from build123d import *

# Parameters (mm, degrees)
BOSS_EXTRUDE1_DEPTH     = 20
FILLET1_R               = 4
SKETCH2_R               = 2.75
CUT_EXTRUDE1_DEPTH      = 1.5
LPATTERN1_COUNT         = 2
LPATTERN1_PITCH         = 30
CUT_EXTRUDE2_DEPTH      = 29.722813233
CUT_EXTRUDE2_DEPTH_BACK = 29.722813233
WRAP1_DEPTH             = 1


# Read off the part's stored shape, not the designer's step: Wrap1
with BuildPart() as part:
    # Sketch1 → Boss-Extrude1 (new body)
    with BuildSketch(Plane(origin=(0, 0, 0), x_dir=(1, 0, 0), z_dir=(0, 1, 0))):
        with BuildLine():
            Line((15, -5), (-15, -5))
            ThreePointArc((-15, -5), (-20, 0), (-15, 5))
            Line((-15, 5), (15, 5))
            ThreePointArc((15, 5), (20, 0), (15, -5))
        make_face()
    extrude(amount=BOSS_EXTRUDE1_DEPTH)

    # Fillet1
    fillet1_edges = [part.edges().sort_by_distance(p)[0] for p in [
        (-20, 20, 0),
        (0, 20, 5),
        (20, 20, 0),
        (0, 20, -5),
    ]]
    fillet(fillet1_edges, radius=FILLET1_R)

    # Sketch2 → Cut-Extrude1 (cut)
    with BuildSketch(Plane.XZ):
        with Locations(Location((-15, 0, 0), (0, 0, 270))):
            Circle(SKETCH2_R)
    cut_extrude1 = extrude(amount=-CUT_EXTRUDE1_DEPTH, mode=Mode.SUBTRACT)

    # LPattern1: Cut-Extrude1 ×2
    with Locations(*[(i * LPATTERN1_PITCH, 0, 0) for i in range(1, LPATTERN1_COUNT)]):
        add(cut_extrude1, mode=Mode.SUBTRACT)

    # Sketch3 → Cut-Extrude2 (cut, two sides: drawn at the far end of the back side and taken through both)
    with BuildSketch(Plane.XY.offset(-CUT_EXTRUDE2_DEPTH_BACK)):
        with BuildLine():
            Line((-5, 23), (5, 23))
            ThreePointArc((5, 23), (8, 20), (5, 17))
            Line((5, 17), (-5, 17))
            ThreePointArc((-5, 17), (-8, 20), (-5, 23))
        make_face()
    extrude(amount=CUT_EXTRUDE2_DEPTH + CUT_EXTRUDE2_DEPTH_BACK, mode=Mode.SUBTRACT)

    # Wrap1 outline → Wrap1 (add)
    with BuildSketch(Plane(origin=(0, 17, 0), x_dir=(1, 0, 0), z_dir=(0, 1, 0))):
        with BuildLine():
            add(Edge.make_bspline(
                [(0.968558604, -2.112404227), (1.023340463, -2.110381468), (1.128135866, -2.106512015), (1.275421614, -2.065066433), (1.40411806, -1.999153831), (1.494113345, -1.918796765), (1.555259283, -1.8377784), (1.600182088, -1.761379971), (1.643056037, -1.669468115), (1.68410688, -1.562162987), (1.724115658, -1.439672484), (1.762787282, -1.301883834), (1.796828359, -1.147944523), (1.819117415, -1.040313742), (1.830738091, -0.984199098)],
                knots=[0, 0, 0, 0, 0.10403341, 0.199011557, 0.288612319, 0.377191825, 0.425797175, 0.481425289, 0.545557079, 0.61863331, 0.699984683, 0.790771883, 0.890916323, 1, 1, 1, 1], degree=3))
            Line((0.968558604, -2.112404227), (-1.502595242, -2.112404227))
            add(Edge.make_bspline(
                [(0.359584245, -0.57875038), (0.287589412, -0.631266446), (0.149119993, -0.732271876), (-0.052040125, -0.874957595), (-0.232151558, -1.010570949), (-0.396984875, -1.13231455), (-0.543079134, -1.243803459), (-0.672030163, -1.343433338), (-0.782764208, -1.43141572), (-0.961872458, -1.579798827), (-1.207220157, -1.798528227), (-1.40469562, -2.00837263), (-1.502595242, -2.112404227)],
                knots=[0, 0, 0, 0, 0.110593572, 0.212707314, 0.306051588, 0.390379305, 0.467018215, 0.534117187, 0.592614819, 0.642525788, 0.822780058, 1, 1, 1, 1], degree=3))
            add(Edge.make_bspline(
                [(2.103173989, 1.329903466), (2.066781163, 1.246346618), (1.99482956, 1.081147874), (1.86047631, 0.847661593), (1.71297016, 0.626020413), (1.571074283, 0.452909604), (1.445054335, 0.315568643), (1.334068385, 0.207346612), (1.208958187, 0.091994137), (1.069166496, -0.030104), (0.913592831, -0.158279882), (0.741560734, -0.29208501), (0.556771712, -0.435146764), (0.42660857, -0.529939289), (0.359584245, -0.57875038)],
                knots=[0, 0, 0, 0, 0.10413489, 0.205883221, 0.307528832, 0.408265615, 0.461433854, 0.520606469, 0.585444086, 0.656004792, 0.732803839, 0.815893726, 0.905198979, 1, 1, 1, 1], degree=3))
            add(Edge.make_bspline(
                [(2.258622707, 2.155223979), (2.256854974, 2.081406691), (2.253395008, 1.936924834), (2.223825952, 1.724789841), (2.174767432, 1.522306219), (2.126875674, 1.393600214), (2.103173989, 1.329903466)],
                knots=[0, 0, 0, 0, 0.261979501, 0.512769921, 0.758869279, 1, 1, 1, 1], degree=3))
            add(Edge.make_bspline(
                [(-0.061890114, 4.14400603), (0.022564629, 4.141920306), (0.18812583, 4.13783155), (0.430620451, 4.112847977), (0.660471364, 4.067558501), (0.878305178, 4.005888588), (1.082018473, 3.923000729), (1.274759097, 3.825795699), (1.453280397, 3.707304776), (1.618929442, 3.573545968), (1.768923738, 3.427244365), (1.900049838, 3.270535022), (2.011299511, 3.105351175), (2.101257211, 2.93081783), (2.172841542, 2.749020464), (2.221753805, 2.558426678), (2.253872753, 2.359840276), (2.257020026, 2.224263519), (2.258622707, 2.155223979)],
                knots=[0, 0, 0, 0, 0.074102612, 0.14526736, 0.21355926, 0.279416432, 0.343556942, 0.406228654, 0.468492489, 0.531146675, 0.592790073, 0.652016559, 0.710119813, 0.767135501, 0.823967905, 0.881147087, 0.939476717, 1, 1, 1, 1], degree=3))
            add(Edge.make_bspline(
                [(-1.906441396, 3.445288081), (-1.848306189, 3.501112989), (-1.732554849, 3.612264359), (-1.538609793, 3.754854821), (-1.330466242, 3.876473687), (-1.105791254, 3.973994027), (-0.866480346, 4.051164268), (-0.611446439, 4.105367467), (-0.341562002, 4.137488539), (-0.156530269, 4.14180053), (-0.061890114, 4.14400603)],
                knots=[0, 0, 0, 0, 0.119107626, 0.23715177, 0.355050392, 0.47498588, 0.598670295, 0.726365388, 0.860041186, 1, 1, 1, 1], degree=3))
            add(Edge.make_bspline(
                [(-2.459326011, 2.031826543), (-2.458122329, 2.10083777), (-2.455751672, 2.236755643), (-2.42704922, 2.435648535), (-2.383831572, 2.625974396), (-2.325084873, 2.808678323), (-2.245799792, 2.981581962), (-2.150493697, 3.146407777), (-2.038697096, 3.303051555), (-1.950794522, 3.397587797), (-1.906441396, 3.445288081)],
                knots=[0, 0, 0, 0, 0.132803649, 0.26155729, 0.386082589, 0.508400008, 0.630401232, 0.751619273, 0.874674186, 1, 1, 1, 1], degree=3))
            add(Edge.make_bspline(
                [(-1.520223447, 0.759390645), (-1.585420599, 0.763118791), (-1.713143024, 0.770422298), (-1.895082142, 0.836934937), (-2.058691576, 0.943915448), (-2.201841078, 1.092044894), (-2.320121913, 1.277705611), (-2.399559254, 1.501224402), (-2.452612405, 1.75530448), (-2.457009968, 1.936432658), (-2.459326011, 2.031826543)],
                knots=[0, 0, 0, 0, 0.110139331, 0.215764983, 0.323707128, 0.438906263, 0.562183724, 0.693638164, 0.838649921, 1, 1, 1, 1], degree=3))
            add(Edge.make_bspline(
                [(-0.613172165, 1.631185517), (-0.616054345, 1.570486701), (-0.621662157, 1.45238594), (-0.671323685, 1.283175242), (-0.754629801, 1.131365188), (-0.869218028, 1.000302814), (-1.00648217, 0.893380798), (-1.162575656, 0.81342959), (-1.336719307, 0.768952542), (-1.458017598, 0.762632021), (-1.520223447, 0.759390645)],
                knots=[0, 0, 0, 0, 0.129242333, 0.251464839, 0.372304265, 0.495878621, 0.620081591, 0.741344555, 0.867352775, 1, 1, 1, 1], degree=3))
            add(Edge.make_bspline(
                [(-1.273428575, 2.371570132), (-1.221111857, 2.356431424), (-1.121681232, 2.327659528), (-0.986315759, 2.264054818), (-0.872118751, 2.188748181), (-0.775565412, 2.103031066), (-0.702763657, 2.001965174), (-0.650977929, 1.888692008), (-0.61737495, 1.763975364), (-0.614599413, 1.676280399), (-0.613172165, 1.631185517)],
                knots=[0, 0, 0, 0, 0.151156851, 0.287281401, 0.413669873, 0.530293514, 0.644009236, 0.756908248, 0.874996313, 1, 1, 1, 1], degree=3))
            add(Edge.make_bspline(
                [(-1.659646524, 2.52701885), (-1.641908981, 2.5134804), (-1.599762076, 2.48131113), (-1.513799429, 2.446453071), (-1.403911325, 2.405291879), (-1.319666952, 2.383519902), (-1.273428575, 2.371570132)],
                knots=[0, 0, 0, 0, 0.159109439, 0.378066483, 0.65864549, 1, 1, 1, 1], degree=3))
            add(Edge.make_bspline(
                [(-1.741377293, 2.725736799), (-1.740702967, 2.705828636), (-1.739402264, 2.667427893), (-1.722346439, 2.613602242), (-1.696843256, 2.565494988), (-1.672067897, 2.539867464), (-1.659646524, 2.52701885)],
                knots=[0, 0, 0, 0, 0.268945253, 0.518766978, 0.758729042, 1, 1, 1, 1], degree=3))
            add(Edge.make_bspline(
                [(-0.509005498, 3.631185517), (-0.593702292, 3.627478268), (-0.757485819, 3.620309328), (-0.992510379, 3.565399378), (-1.204920463, 3.4708981), (-1.388970755, 3.342097951), (-1.54050767, 3.195942921), (-1.655393233, 3.044422755), (-1.727025811, 2.886507887), (-1.736695124, 2.778188345), (-1.741377293, 2.725736799)],
                knots=[0, 0, 0, 0, 0.151816317, 0.293576777, 0.429964406, 0.566304914, 0.694365033, 0.806085808, 0.906100976, 1, 1, 1, 1], degree=3))
            add(Edge.make_bspline(
                [(0.617597066, 2.220929107), (0.616798314, 2.277062503), (0.615251229, 2.385786079), (0.599863671, 2.542997259), (0.579004071, 2.690242583), (0.544058374, 2.826348498), (0.504153512, 2.954009696), (0.449772713, 3.069509609), (0.389899195, 3.176431124), (0.318093883, 3.271087373), (0.240513737, 3.356936451), (0.152380296, 3.428872442), (0.059506725, 3.491963217), (-0.040243661, 3.543993611), (-0.147906764, 3.581901434), (-0.261368703, 3.611540097), (-0.38306343, 3.626855058), (-0.466235221, 3.629714881), (-0.509005498, 3.631185517)],
                knots=[0, 0, 0, 0, 0.082284271, 0.159374645, 0.231497254, 0.300083139, 0.36523236, 0.427274673, 0.486932074, 0.544586116, 0.60112786, 0.656190593, 0.710940404, 0.765594865, 0.820607428, 0.877984079, 0.93725451, 1, 1, 1, 1], degree=3))
            add(Edge.make_bspline(
                [(0.205738091, 0.635993209), (0.238640814, 0.700768661), (0.303861654, 0.829168655), (0.385865127, 1.026897746), (0.459663901, 1.22391557), (0.516579645, 1.422967903), (0.561905142, 1.621957205), (0.593823909, 1.82108009), (0.613938148, 2.020726724), (0.616375849, 2.154108657), (0.617597066, 2.220929107)],
                knots=[0, 0, 0, 0, 0.131745637, 0.261150462, 0.388067803, 0.513189353, 0.636374668, 0.758087597, 0.878808958, 1, 1, 1, 1], degree=3))
            add(Edge.make_bspline(
                [(-1.116377293, -1.107596534), (-1.03496234, -1.013767374), (-0.878016077, -0.832889839), (-0.655626445, -0.569536189), (-0.456135085, -0.32390871), (-0.280159151, -0.096566641), (-0.125247461, 0.111659158), (0.00577288, 0.302221735), (0.116680709, 0.473318508), (0.177475044, 0.584367138), (0.205738091, 0.635993209)],
                knots=[0, 0, 0, 0, 0.170005554, 0.327725258, 0.471696803, 0.603008639, 0.721148947, 0.826797124, 0.919478664, 1, 1, 1, 1], degree=3))
            add(Edge.make_bspline(
                [(-2.664454216, -3.057917047), (-2.628698989, -3.000910883), (-2.55158858, -2.877970296), (-2.41479269, -2.688825323), (-2.259314405, -2.474715573), (-2.074551732, -2.243606397), (-1.870318919, -1.988170585), (-1.640593125, -1.712928149), (-1.387471618, -1.416348269), (-1.20904993, -1.213142224), (-1.116377293, -1.107596534)],
                knots=[0, 0, 0, 0, 0.080973991, 0.174630064, 0.280853316, 0.39944862, 0.530692677, 0.674513651, 0.830941638, 1, 1, 1, 1], degree=3))
            Line((-2.664454216, -3.057917047), (-2.664454216, -3.548301662))
            Line((-2.664454216, -3.548301662), (2.156058604, -3.548301662))
            Line((2.156058604, -3.548301662), (2.361186809, -0.984199098))
            Line((2.361186809, -0.984199098), (1.830738091, -0.984199098))
        make_face()
    extrude(amount=WRAP1_DEPTH)


solid = part.part
Work out the finished part from the listing and answer in its coordinate system (mm). A direction names the side the tool comes from. Coordinates: 2 decimals unless noted, no trailing zeros. Loops run counter-clockwise (first coordinate to the right, second up) from the corner with the lowest first, then second, coordinate; pieces in that order, holes last. Notation, with made-up numbers: (80, 20) -> (132, 20) arc R16 ccw to (132, 35) -> close; hole circle Ø10 at (-33.75, -20.5). An arc over 180 degrees is marked (long way). Answer as CSV lines item,"result".
1) The part is cut by section C-C (x = 13.5). Give the vertices of the cut face in (y, z), and give its area (3 significant figures).
A:
outline,"(0, -5) -> (16, -5) arc R4 ccw to (20, -1) -> (20, 1) arc R4 ccw to (16, 5) -> (0, 5) -> (0, 2.3) -> (1.5, 2.3) -> (1.5, -2.3) -> (0, -2.3) -> close"
area,"186 mm²"
2) Flat-ended cylindrical pins translate along their axes: pin 1 (0.8 mm diameter, centred on x = -0.5, y = 17.5, fed in from -Z); pin 2 (3.5 mm diameter, centred on x = 15, z = 0, fed in from -Y); pin 3 (1.5 mm diameter, centred on y = 8.5, z = -2, fed in from -X). Find the tip coordinate at first contact, or state that the pin passes through.
A:
pin 1,"stops at z = -4.14"
pin 2,"stops at y = 1.5"
pin 3,"stops at x = -19.84"
3) Straight lines are drawn through the part: probe 1 along X at (y, z) = (1.1, 0); probe 2 along Y at (x, z) = (3.5, -3.25); probe 3 along X at (y, z) = (11.75, -0.25). For each, find the intervals that lie inside material, in ascending order.
A:
probe 1,"x = -20 to -17.75, -12.25 to 12.25, 17.75 to 20"
probe 2,"y = 0 to 17"
probe 3,"x = -19.99 to 19.99"
4) For a pull along X with two mould halves and no side action, classify faces 6 (the face through (2.257, 17.493, 2.284)), 7 (the face through (0, 0, 0)), 8 (the face through (20, 8, 0)) as released by +X, released by -X, zero draft, split by the parting line, or undercut.
A:
face 6,"undercut"
face 7,"zero draft"
face 8,"released by +X"
5) The part is cut by section A-A (x = -5.5). Give the vertices of the cut face in (y, z).
A:
outline,"(0, -5) -> (16, -5) arc R4 ccw to (17.04, -4.86) -> (17.04, 4.86) arc R4 ccw to (16, 5) -> (0, 5) -> close"
6) The part is cut by section D-D (x = 7.5). Give the vertices of the cut face in (y, z), and give its area (3 significant figures).
A:
outline,"(0, -5) -> (16, -5) arc R4 ccw to (18.34, -4.24) -> (18.34, 4.24) arc R4 ccw to (16, 5) -> (0, 5) -> close"
area,"182 mm²"
7) The part is cut by section B-B (y = 2.25). Give the vertices of the cut face in (x, z), and give its area (3 significant figures).
A:
outline,"(-15, -5) -> (15, -5) arc R5 ccw to (15, 5) -> (-15, 5) arc R5 ccw to start"
area,"379 mm²"
8) For faces 1 (the face through (-0.21, 16.3, 4.99)), 2 (the face through (7.14, 17.9, -0.07)), 3 (the face through (-0.3, 17.5, 3.548)), 4 (the face through (15, 1.5, 0)), 5 (the face through (12, 20, 0)), determine the directions among +Z, -Z, +X, -X, +Y, -Y from which every point of the face is accessible in a straight line to the end or side of a thin tool.
A:
face 1,"+Z, +X, -X, +Y"
face 2,"+Z, -Z, +Y"
face 3,"+Z, +Y"
face 4,"-Y"
face 5,"+Z, -Z, +X, -X, +Y"
